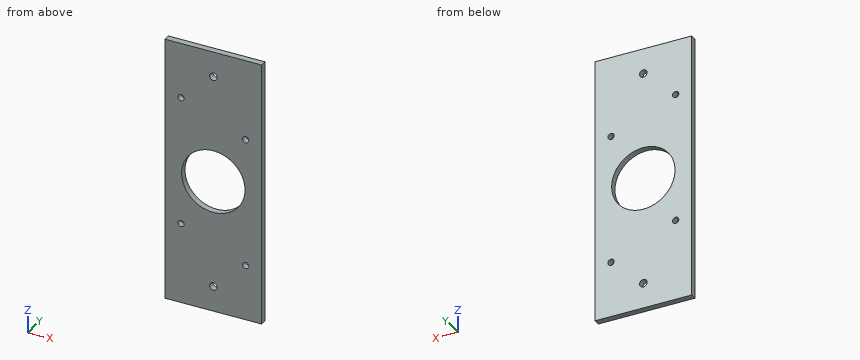
```python
from build123d import *

# Parameters (mm, degrees)
SKETCH1_W           = 76
SKETCH1_H           = 210
SKETCH1_R           = 3
SKETCH1_R_2         = 2.5
SKETCH1_R_3         = 25
BOSS_EXTRUDE1_DEPTH = 5


with BuildPart() as part:
    # Sketch1 → Boss-Extrude1 (new body)
    with BuildSketch(Plane(origin=(0, 0, 0), x_dir=(1, 0, 0), z_dir=(0, 1, 0))):
        with Locations((-31.026205917, -6.39064)):
            Rectangle(SKETCH1_W, SKETCH1_H)
        with Locations((-31.026205917, 78.60936)):
            Circle(SKETCH1_R, mode=Mode.SUBTRACT)
        with Locations((-31.026205917, -91.39064)):
            Circle(SKETCH1_R, mode=Mode.SUBTRACT)
        with Locations((-56.526205917, 34.60936)):
            Circle(SKETCH1_R_2, mode=Mode.SUBTRACT)
        with Locations((-5.526205917, 54.60936)):
            Circle(SKETCH1_R_2, mode=Mode.SUBTRACT)
        with Locations((-56.526205917, -67.39064)):
            Circle(SKETCH1_R_2, mode=Mode.SUBTRACT)
        with Locations((-5.526205917, -47.39064)):
            Circle(SKETCH1_R_2, mode=Mode.SUBTRACT)
        with Locations((-31.026205917, -6.39064)):
            Circle(SKETCH1_R_3, mode=Mode.SUBTRACT)
    extrude(amount=BOSS_EXTRUDE1_DEPTH)


solid = part.part
```
Can you work these out from the model? Positions are in its coordinate system, mm. Round coordinates to 2 decimals unless told otherwise and drop trailing zeros. Order: outer loops, then holes, each group sorted by start corner. A loop starts at its lowest first (then second) coordinate and runs counter-clockwise, first axis right, second up.
(1) If we section it at B-B (y = 4): Please give me the cut outline in (x, z).
Results are:
outline: (-69.03, -98.61) - (6.97, -98.61) - (6.97, 111.39) - (-69.03, 111.39) - close; hole circle Ø5 at (-56.53, -34.61); hole circle Ø5 at (-56.53, 67.39); hole circle Ø50 at (-31.03, 6.39); hole circle Ø6 at (-31.03, -78.61); hole circle Ø6 at (-31.03, 91.39); hole circle Ø5 at (-5.53, -54.61); hole circle Ø5 at (-5.53, 47.39)
(2) If we section it at C-C (x = -18): Please give me the cut outline in (y, z).
Results are:
outline: (0, -98.61) - (5, -98.61) - (5, -14.95) - (0, -14.95) - close; (0, 27.73) - (5, 27.73) - (5, 111.39) - (0, 111.39) - close
(3) If I drill on L1, parallel to Z at x = -58, y = 3.7; L2, parallel to Z at x = -30, y = 4.3; L3, parallel to Z at x = -47.5, y = 4, over which ranges is the centre line in solid material (lowest first)?
Results are:
L1: z = -98.61 to -36.63, -32.59 to 65.37, 69.41 to 111.39
L2: z = -98.61 to -81.43, -75.79 to -18.59, 31.37 to 88.57, 94.21 to 111.39
L3: z = -98.61 to -12.41, 25.2 to 111.39
(4) I'm going to push a flat-ended pin straight in: pin 1 (10 mm diameter, centred on x = -7, z = -48, fed in from -Y). Where does the tip first touch, or does it pass through?
Results are:
pin 1: stops at y = 0
(5) If we section it at A-A (z = 26.5): Please give me the cut outline in (x, y).
Results are:
outline: (-69.03, 0) - (-45.88, 0) - (-45.88, 5) - (-69.03, 5) - close; (-16.17, 0) - (6.97, 0) - (6.97, 5) - (-16.17, 5) - close
